from build123d import *

# Parameters (mm, degrees)
F1_DEPTH = 23
F0_R     = 1.05
F0_W     = 22.4
F0_H     = 12
F2_DEPTH = 3
F4_D     = 3.3
F4_DEPTH = 12
F4_TIP   = 0.9914200214
F5_W     = 5.6
F5_H     = 2.5
F7_DEPTH = 6.8
F6_W     = 5.6
F6_H     = 2.5
F8_DEPTH = 6.8
F9_R     = 5
F10_R    = 0.5


with BuildPart() as f1:
    # F0 (on Top) → F1 (new body)
    with BuildSketch(Plane.XY):
        with BuildLine():
            Line((-10.925, 11), (-8.5, 11))
            Line((-8.5, 11), (-8.5, 15))
            Line((-8.5, 15), (-16.5, 15))
            Line((-16.5, 15), (-16.5, 11))
            Line((-16.5, 11), (-14.075, 11))
            ThreePointArc((-14.075, 11), (-12.5, 12.575), (-10.925, 11))
        make_face()
        with BuildLine():
            Line((-14.075, 11), (-10.925, 11))
            ThreePointArc((-10.925, 11), (-12.5, 12.575), (-14.075, 11))
        make_face()
        with BuildLine():
            ThreePointArc((-14.075, 11), (-12.5, 9.425), (-10.925, 11))
            Line((-10.925, 11), (-14.075, 11))
        make_face()
        with BuildLine():
            Line((-8.5, 7), (-8.5, 11))
            Line((-8.5, 11), (-10.925, 11))
            ThreePointArc((-10.925, 11), (-12.5, 9.425), (-14.075, 11))
            Line((-14.075, 11), (-16.5, 11))
            Line((-16.5, 11), (-16.5, 7))
            Line((-16.5, 7), (-8.5, 7))
        make_face()
    extrude(amount=-F1_DEPTH)



with BuildPart() as f1b:
    # F0 (on Top) → F1, piece 2 (new body)
    with BuildSketch(Plane.XY):
        with BuildLine():
            Line((14.075, 11), (16.5, 11))
            Line((16.5, 11), (16.5, 15))
            Line((16.5, 15), (8.5, 15))
            Line((8.5, 15), (8.5, 11))
            Line((8.5, 11), (10.925, 11))
            ThreePointArc((10.925, 11), (12.5, 12.575), (14.075, 11))
        make_face()
        with BuildLine():
            Line((10.925, 11), (14.075, 11))
            ThreePointArc((14.075, 11), (12.5, 12.575), (10.925, 11))
        make_face()
        with BuildLine():
            ThreePointArc((10.925, 11), (12.5, 9.425), (14.075, 11))
            Line((14.075, 11), (10.925, 11))
        make_face()
        with BuildLine():
            Line((8.5, 7), (16.5, 7))
            Line((16.5, 7), (16.5, 11))
            Line((16.5, 11), (14.075, 11))
            ThreePointArc((14.075, 11), (12.5, 9.425), (10.925, 11))
            Line((10.925, 11), (8.5, 11))
            Line((8.5, 11), (8.5, 7))
        make_face()
    extrude(amount=-F1_DEPTH)


with BuildPart() as f1c:
    # F0 (on Top) → F1, piece 3 (new body)
    with BuildSketch(Plane.XY):
        with BuildLine():
            Line((-10.925, -11), (-8.5, -11))
            Line((-8.5, -11), (-8.5, -7))
            Line((-8.5, -7), (-16.5, -7))
            Line((-16.5, -7), (-16.5, -11))
            Line((-16.5, -11), (-14.075, -11))
            ThreePointArc((-14.075, -11), (-12.5, -9.425), (-10.925, -11))
        make_face()
        with BuildLine():
            Line((-14.075, -11), (-10.925, -11))
            ThreePointArc((-10.925, -11), (-12.5, -9.425), (-14.075, -11))
        make_face()
        with BuildLine():
            ThreePointArc((-14.075, -11), (-12.5, -12.575), (-10.925, -11))
            Line((-10.925, -11), (-14.075, -11))
        make_face()
        with BuildLine():
            Line((-8.5, -15), (-8.5, -11))
            Line((-8.5, -11), (-10.925, -11))
            ThreePointArc((-10.925, -11), (-12.5, -12.575), (-14.075, -11))
            Line((-14.075, -11), (-16.5, -11))
            Line((-16.5, -11), (-16.5, -15))
            Line((-16.5, -15), (-8.5, -15))
        make_face()
    extrude(amount=-F1_DEPTH)


with BuildPart() as f1d:
    # F0 (on Top) → F1, piece 4 (new body)
    with BuildSketch(Plane.XY):
        with BuildLine():
            Line((10.925, -11), (14.075, -11))
            ThreePointArc((14.075, -11), (12.5, -9.425), (10.925, -11))
        make_face()
        with BuildLine():
            ThreePointArc((10.925, -11), (12.5, -12.575), (14.075, -11))
            Line((14.075, -11), (10.925, -11))
        make_face()
        with BuildLine():
            Line((14.075, -11), (16.5, -11))
            Line((16.5, -11), (16.5, -7))
            Line((16.5, -7), (8.5, -7))
            Line((8.5, -7), (8.5, -11))
            Line((8.5, -11), (10.925, -11))
            ThreePointArc((10.925, -11), (12.5, -9.425), (14.075, -11))
        make_face()
        with BuildLine():
            Line((16.5, -15), (16.5, -11))
            Line((16.5, -11), (14.075, -11))
            ThreePointArc((14.075, -11), (12.5, -12.575), (10.925, -11))
            Line((10.925, -11), (8.5, -11))
            Line((8.5, -11), (8.5, -15))
            Line((8.5, -15), (16.5, -15))
        make_face()
    extrude(amount=-F1_DEPTH)


with BuildPart() as f1_1:
    add(f1.part)

    add(f1b.part)  # F2 merges F1b

    add(f1c.part)  # F2 merges F1c

    add(f1d.part)  # F2 merges F1d
    # F0 (on Top) → F2 (join)
    with BuildSketch(Plane.XY):
        Polygon((8.5, -7), (16.5, -7), (16.5, 7), (8.5, 7), (8.5, 11), (-8.5, 11), (-8.5, 7), (-16.5, 7), (-16.5, -7), (-8.5, -7), (-8.5, -11), (8.5, -11), align=None)
        with Locations((-13.875, 0)):
            Circle(F0_R, mode=Mode.SUBTRACT)
        Rectangle(F0_W, F0_H, mode=Mode.SUBTRACT)
        with Locations((13.875, 0)):
            Circle(F0_R, mode=Mode.SUBTRACT)
    extrude(amount=-F2_DEPTH)

    # F4
    with Locations(Plane(origin=(0, 0, -23), x_dir=(1, 0, 0), z_dir=(0, 0, -1))):
        with Locations((-12.5, 11), (12.5, 11), (-12.5, -11), (12.5, -11)):
            Hole(F4_D / 2, depth=F4_DEPTH)
            with Locations((0, 0, -(F4_DEPTH + F4_TIP / 2))):  # 118° drill point
                Cone(0, F4_D / 2, F4_TIP, mode=Mode.SUBTRACT)

    # F5 (on face) → F7 (cut)
    with BuildSketch(Plane.XZ.offset(15)):
        with Locations((-12.5, -18.25)):
            Rectangle(F5_W, F5_H)
        with Locations((12.5, -18.25)):
            Rectangle(F5_W, F5_H)
    extrude(amount=-F7_DEPTH, mode=Mode.SUBTRACT)

    # F6 (on face) → F8 (cut)
    with BuildSketch(Plane(origin=(0, 15, 0), x_dir=(-1, 0, 0), z_dir=(0, 1, 0))):
        with Locations((-12.5, -18.25)):
            Rectangle(F6_W, F6_H)
        with Locations((12.5, -18.25)):
            Rectangle(F6_W, F6_H)
    extrude(amount=-F8_DEPTH, mode=Mode.SUBTRACT)

    # F9
    f9_edges = [f1_1.edges().sort_by_distance(p)[0] for p in [
        (12.5, 15, 0),
        (-12.5, -15, 0),
    ]]
    fillet(f9_edges, radius=F9_R)

    # F10
    f10_edges = [f1_1.edges().sort_by_distance(p)[0] for p in [
        (16.5, -15, -14),
        (16.5, -7, -13),
        (-8.5, -15, -14),
        (16.5, 7, -13),
        (-16.5, 15, -14),
        (-8.5, 15, -14),
        (8.5, 15, -14),
        (8.5, -7, -13),
        (8.5, 7, -13),
        (-8.5, 7, -13),
        (-8.5, -7, -13),
        (-16.5, 7, -13),
        (-16.5, -7, -13),
        (8.5, -15, -14),
    ]]
    fillet(f10_edges, radius=F10_R)


solid = f1_1.part
Read the model definition and answer for the solid it produces. Units are mm, in the model's axes. A direction names the side the tool comes from. Round coordinates to 2 decimals unless told otherwise and drop trailing zeros. Loops run counter-clockwise (first coordinate to the right, second up) from the corner with the lowest first, then second, coordinate; pieces in that order, holes last.
Q1. Section C-C on y = -5 is taken. Write down the section's boundary in (x, z).
Q2. Consider probe 1 along X at (y, z) = (11, -22.1); probe 2 along Y at (x, z) = (-12.5, -14.55); probe 3 along X at (y, z) = (13, -19.75). Determine where each line is inside the solid, lowest interval first.
Q3. Each of these flat-tipped pins is pushed along its axis until it touches: pin 1 (3 mm diameter, centred on x = -3.5, z = -1, fed in from +Y); pin 2 (2.5 mm diameter, centred on x = 12.5, y = 11, fed in from -Z); pin 3 (3 mm diameter, centred on x = -12, y = -12.5, fed in from +Z); pin 4 (1.7 mm diameter, centred on x = 13.875, y = 0, fed in from -Z). Where does it stop, or does it pass through?
Q4. Determine the mould class of faces 5 (the face through (15.3, 12, -18)), 6 (the face through (-13, 7, -13)), 7 (the face through (10.7, 11.1, -23)), 8 (the face through (13, 13, -19.5)) for opening direction Z: released by +Z, released by -Z, zero draft, split by the parting line, or undercut.
Q5. Section B-B on x = -5.5 is taken. Write down the section's boundary in (y, z), and give its area (3 significant figures).
Q6. Section D-D on z = -4.5 is taken. Give the number of separate pieces and of enclosed holes in the cut face, and give its area (3 significant figures).
Q7. Section A-A on y = 0 is taken. Write down the section's boundary in (x, z) (3 decimals), and give its area (3 significant figures).
Q8. Which of the six approach directions +Z, -Z, +X, -X, +Y, -Y give full straight-line access (tool end or side, diameter ignored) to faces 1 (the face through (-14.024, -10.368, -13.958)), 2 (the face through (-15.3, 12, -18)), 3 (the face through (-12, -7, -13)), 4 (the face through (0.224, -10.381, -0.015))?
Output:
1. outline: (-16.5, -3) - (-11.2, -3) - (-11.2, 0) - (-16, 0) arc R0.5 ccw to (-16.5, -0.5) - close; (11.2, -3) - (16.5, -3) - (16.5, -0.5) arc R0.5 ccw to (16, 0) - (11.2, 0) - close
2. probe 1: x = -16.5 to -14.15, -10.85 to -8.5, 8.5 to 10.85, 14.15 to 16.5
2. probe 2: y = -15 to -12.65, -9.35 to -7, 7 to 9.35, 12.65 to 15
2. probe 3: x = -16.5 to -8.5, 8.5 to 16.5
3. pin 1: stops at y = 11
3. pin 2: stops at z = -10.76
3. pin 3: stops at z = -0.1
3. pin 4: passes through
4. face 5: undercut
4. face 6: zero draft
4. face 7: released by -Z
4. face 8: undercut
5. outline: (-11, -3) - (-6, -3) - (-6, 0) - (-10, 0) arc R5 ccw to (-11, -0.1) - close; (6, -3) - (11, -3) - (11, -0.1) arc R5 ccw to (10, 0) - (6, 0) - close
5. area: 29.9 mm2
6. separate pieces: 4
6. enclosed holes: 0
6. area: 254 mm2
7. outline: (-16.5, -3) - (-14.925, -3) - (-14.925, 0) - (-16, 0) arc R0.5 ccw to (-16.5, -0.5) - close; (-12.825, -3) - (-11.2, -3) - (-11.2, 0) - (-12.825, 0) - close; (11.2, -3) - (12.825, -3) - (12.825, 0) - (11.2, 0) - close; (14.925, -3) - (16.5, -3) - (16.5, -0.5) arc R0.5 ccw to (16, 0) - (14.925, 0) - close
7. area: 19.1 mm2
8. face 1: -Z
8. face 2: +Y
8. face 3: -Z, +X, -X
8. face 4: +Z, +X, -X, -Y
